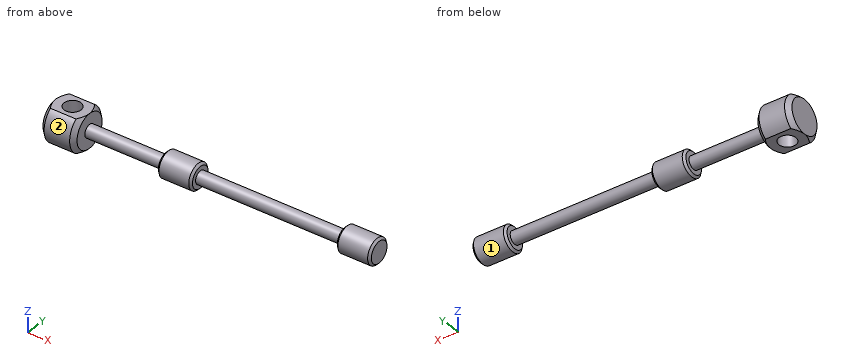
from build123d import *

# Parameters (mm, degrees)
SKETCH1_R               = 1.5
BOSS_EXTRUDE1_DEPTH     = 50
SKETCH2_R               = 3
BOSS_EXTRUDE2_DEPTH     = 8
CHAMFER1_SIZE           = 0.5
SKETCH3_R               = 3
BOSS_EXTRUDE4_DEPTH     = 8
CHAMFER2_SIZE           = 0.5
SKETCH5_R               = 1.5
BOSS_EXTRUDE5_DEPTH     = 26
SKETCH6_R               = 5
BOSS_EXTRUDE6_DEPTH     = 8
SKETCH7_R               = 2
CUT_EXTRUDE1_DEPTH      = 6
CUT_EXTRUDE1_DEPTH_BACK = 6
CHAMFER3_SIZE           = 1
CUT_EXTRUDE2_DEPTH      = 1
CUT_EXTRUDE2_DEPTH_BACK = 77


with BuildPart() as part:
    # Sketch1 → Boss-Extrude1 (new body)
    with BuildSketch(Plane(origin=(0, 0, 0), x_dir=(0, 0, -1), z_dir=(1, 0, 0))):
        Circle(SKETCH1_R)
    extrude(amount=BOSS_EXTRUDE1_DEPTH)

    # Sketch2 → Boss-Extrude2 (add)
    with BuildSketch(Plane(origin=(50, 0, 0), x_dir=(0, 0, -1), z_dir=(1, 0, 0))):
        Circle(SKETCH2_R)
    extrude(amount=-BOSS_EXTRUDE2_DEPTH)

    # Chamfer1
    chamfer1_edges = [part.edges().sort_by_distance(p)[0] for p in [
        (42, 0, 3),
        (50, 0, 3),
    ]]
    chamfer(chamfer1_edges, length=CHAMFER1_SIZE)

    # Sketch3 → Boss-Extrude4 (add)
    with BuildSketch(Plane.ZY):
        Circle(SKETCH3_R)
    extrude(amount=-BOSS_EXTRUDE4_DEPTH)

    # Chamfer2
    chamfer2_edges = [part.edges().sort_by_distance(p)[0] for p in [
        (8, 0, -3),
        (0, 0, -3),
    ]]
    chamfer(chamfer2_edges, length=CHAMFER2_SIZE)

    # Sketch5 → Boss-Extrude5 (add)
    with BuildSketch(Plane.ZY):
        Circle(SKETCH5_R)
    extrude(amount=BOSS_EXTRUDE5_DEPTH)

    # Sketch6 → Boss-Extrude6 (add)
    with BuildSketch(Plane.ZY.offset(26)):
        Circle(SKETCH6_R)
    extrude(amount=-BOSS_EXTRUDE6_DEPTH)

    # Sketch7 → Cut-Extrude1 (cut, two sides)
    with BuildSketch(Plane.XY) as cut_extrude1_sk:
        with Locations((-22, 0)):
            Circle(SKETCH7_R)
    extrude(amount=CUT_EXTRUDE1_DEPTH, mode=Mode.SUBTRACT)
    extrude(cut_extrude1_sk.sketch, amount=-CUT_EXTRUDE1_DEPTH_BACK, mode=Mode.SUBTRACT)

    # Chamfer3
    chamfer3_edges = [part.edges().sort_by_distance(p)[0] for p in [
        (-18, 0, -5),
        (-26, 0, -5),
    ]]
    chamfer(chamfer3_edges, length=CHAMFER3_SIZE)

    # Sketch8 → Cut-Extrude2 (cut, two sides)
    with BuildSketch(Plane.ZY.offset(26)) as cut_extrude2_sk:
        with BuildLine():
            Line((-4, 4), (-4, -4))
            ThreePointArc((-4, -4), (-5.656854249, 0), (-4, 4))
        make_face()
        with BuildLine():
            Line((4, 4), (4, -4))
            ThreePointArc((4, -4), (5.656854249, 0), (4, 4))
        make_face()
    extrude(amount=CUT_EXTRUDE2_DEPTH, mode=Mode.SUBTRACT)
    extrude(cut_extrude2_sk.sketch, amount=-CUT_EXTRUDE2_DEPTH_BACK, mode=Mode.SUBTRACT)


solid = part.part
Part model, mm, in its own coordinate system. Face numbers are marked on the shaded views. A direction names the side the tool comes from. Give positions to 0.01 mm unless a question says otherwise; leave off trailing zeros. Loops run counter-clockwise (first coordinate to the right, second up) from the corner with the lowest first, then second, coordinate; pieces in that order, holes last. Notation, with made-up numbers: M 74.25,65 L 104.25,65 A18 ccw 104.25,78 Z; hole C 43,50.5 d11. An arc over 180 degrees is marked long. Put each result on its own line as item: value. Start each with the question number.
1) Flat gauge pins, fed straight in: pin 1 (4 mm diameter, centred on x = 32, z = -1.5, fed in from -Y); pin 2 (3 mm diameter, centred on x = -5.5, y = 1.5, fed in from +Z); pin 3 (3.5 mm diameter, centred on x = -22, y = 0, fed in from +Z); pin 4 (1 mm diameter, centred on x = 13.5, z = 1.5, fed in from -Y). Where does each tip first touch, or does it go through?
2) Saw through at A-A (x = -22). List the corners of the cut face in (y, z).
3) Probe probe 1 along X at (y, z) = (0, -0.5); probe 2 along Y at (x, z) = (-22, -0.25); probe 3 along X at (y, z) = (1, -1.25). List the from-to ranges inside material, lowest first.
4) Saw through at C-C (x = 19). List the corners of the cut face in (y, z).
5) Saw through at D-D (x = 1.5). List the corners of the cut face in (y, z).
6) 3-axis set-ups, long thin cutter, end or side, ignore diameter. For the marked faces 1 and 2: which of +Z, -Z, +X, -X, +Y, -Y reach the whole face in a straight line?
Numbers:
1. pin 1: y = -1.5
1. pin 2: z = 1.5
1. pin 3: through
1. pin 4: y = -1.12
2. outline: M -3,-4 L -2,-4 L -2,4 L -3,4 A5 ccw Z; M 2,-4 L 3,-4 A5 ccw 3,4 L 2,4 Z
3. probe 1: -26 to -24, -20 to 50
3. probe 2: -4.99 to -2, 2 to 4.99
3. probe 3: -26 to -23.73, -20.27 to -18, 0 to 8, 42 to 50
4. outline: C 0,0 d3
5. outline: C 0,0 d6
6. face 1: +X
6. face 2: +X, -X, -Y
